Verification items for this drawing (mm, ordinates from the low corner). Round coordinates to 2 decimals unless told otherwise and drop trailing zeros. Order: outer loops, then holes, each group sorted by start corner. A loop starts at its lowest first (then second) coordinate and runs counter-clockwise, first axis right, second up. Notation, with made-up numbers: (51.25, 8.5) - (101.25, 8.5) arc R23 ccw to (101.25, 20.5) - close; hole circle Ø9 at (22, 19.25). An arc over 180 degrees is marked (long way). Return JSON: item names as keys, results as strings. Group by question number.
Q1. Gauge pin test, flat ends, axial feed: pin 1 Ø1.5 at (x, y) = (29, 1.5) entering from -Z; pin 2 Ø1 at (y, z) = (0.5, 5.5) entering from +X; pin 3 Ø6 at (x, z) = (9.5, 14) entering from -Y; pin 4 Ø0.9 at (y, z) = (2, 23.5) entering from -X. Record the tip position at first contact, or that the pin passes through.
Q2. Sectioned sample at B-B, the plane x = 15.5. Record the cut outline in (y, z), then the cut area to 3 significant figures.
Q3. Sectioned sample at D-D, the plane z = 4.5. Record the cut outline in (x, y), then the cut area to 3 significant figures.
Q4. Sectioned sample at A-A, the plane z = 27. Record the cut outline in (x, y), then the cut area to 3 significant figures.
Q5. Sectioned sample at C-C, the plane y = 1.7. Record the cut outline in (x, z).
Q6. Material ranges on line 1 along X through (y, z) = (0.65, 27); line 2 along Z through (x, y) = (15.5, 0.8); line 3 along Z through (x, y) = (29, 2.3), recorded low to high.
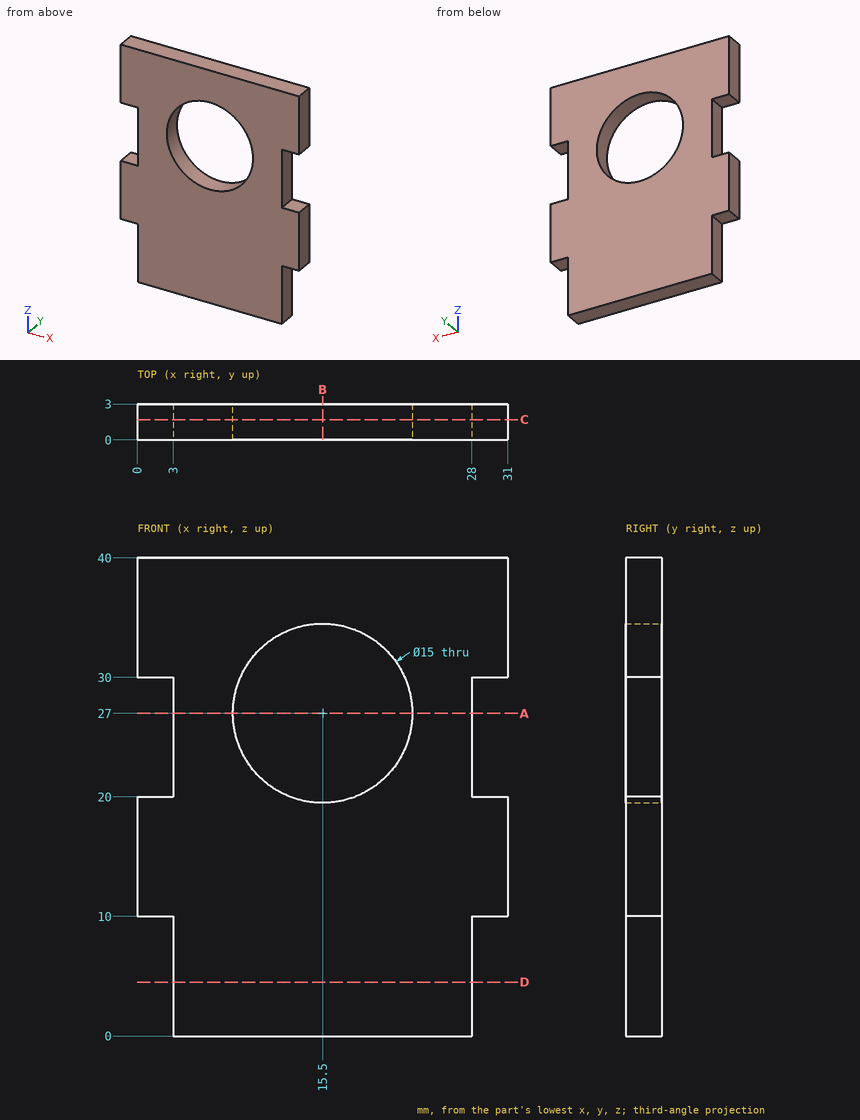
Reply:
{
 "1": {"pin 1": "z = 10", "pin 2": "x = 28", "pin 3": "y = 0", "pin 4": "x = 3"},
 "2": {"outline": "(0, 0) - (3, 0) - (3, 19.5) - (0, 19.5) - close; (0, 34.5) - (3, 34.5) - (3, 40) - (0, 40) - close", "area": "75.0 mm^2"},
 "3": {"outline": "(3, 0) - (28, 0) - (28, 3) - (3, 3) - close", "area": "75.0 mm^2"},
 "4": {"outline": "(3, 0) - (8, 0) - (8, 3) - (3, 3) - close; (23, 0) - (28, 0) - (28, 3) - (23, 3) - close", "area": "30.0 mm^2"},
 "5": {"outline": "(0, 10) - (3, 10) - (3, 0) - (28, 0) - (28, 10) - (31, 10) - (31, 20) - (28, 20) - (28, 30) - (31, 30) - (31, 40) - (0, 40) - (0, 30) - (3, 30) - (3, 20) - (0, 20) - close; hole circle Ø15 at (15.5, 27)"},
 "6": {"line 1": "3 to 8, 23 to 28", "line 2": "0 to 19.5, 34.5 to 40", "line 3": "10 to 20, 30 to 40"}
}
